Read the model definition and answer for the solid it produces. Units are mm, in the model's axes. A direction names the side the tool comes from. Coordinates: 2 decimals unless noted, no trailing zeros. Loops run counter-clockwise (first coordinate to the right, second up) from the corner with the lowest first, then second, coordinate; pieces in that order, holes last. Notation, with made-up numbers: (13, 56) - (32, 56) arc R21 cw to (32, 85) - close; hole circle Ø7 at (4, -30). An arc over 180 degrees is marked (long way). Use one line per item in the form item = value.
from build123d import *

# Parameters (mm, degrees)
SKETCH2_R           = 2.413
BOSS_EXTRUDE1_DEPTH = 57.15
CUT_EXTRUDE1_DEPTH  = 1.778
CHAMFER1_SIZE       = 0.428942381
FILLET1_R           = 0.381


with BuildPart() as part:
    # Sketch1 → Revolve1 (revolve)
    with BuildSketch(Plane.XZ):
        with BuildLine():
            Line((2.29235, 0), (0, 0))
            Line((0, 0), (0, -2.5654))
            Line((0, -2.5654), (4.5847, -2.5654))
            Line((4.5847, -2.5654), (4.5847, -2.0574))
            ThreePointArc((4.5847, -2.0574), (3.589105441, -0.860923645), (2.29235, 0))
        make_face()
    revolve(axis=Axis((0, 0, 0), (0, 0, -1)))

    # Sketch2 → Boss-Extrude1 (add)
    with BuildSketch(Plane(origin=(0, 0, -2.5654), x_dir=(-1, 0, 0), z_dir=(0, 0, -1))):
        Circle(SKETCH2_R)
    extrude(amount=BOSS_EXTRUDE1_DEPTH)

    # Sketch3 → Cut-Extrude1 (cut)
    with BuildSketch(Plane.XY):
        Polygon((1.5875, -0.916543552), (1.5875, 0.916543552), (0, 1.833087105), (-1.5875, 0.916543552), (-1.5875, -0.916543552), (0, -1.833087105), align=None)
    extrude(amount=-CUT_EXTRUDE1_DEPTH, mode=Mode.SUBTRACT)

    # Sketch4 → Cut-Revolve1 (revolve, cut)
    with BuildSketch(Plane.XZ):
        Polygon((1.5875, -1.778), (0, -1.778), (0, -2.694543552), align=None)
    revolve(axis=Axis((0, 0, -1.778), (0, 0, -1)), mode=Mode.SUBTRACT)

    # Chamfer1
    chamfer1_edges = [part.edges().sort_by_distance(p)[0] for p in [
        (2.413, 0, -59.7154),
    ]]
    chamfer(chamfer1_edges, length=CHAMFER1_SIZE)

    # Fillet1
    fillet1_edges = [part.edges().sort_by_distance(p)[0] for p in [
        (2.413, 0, -2.5654),
    ]]
    fillet(fillet1_edges, radius=FILLET1_R)


solid = part.part
Item 1: Find the intervals of material crossed by L1, parallel to Y at x = -0.75, z = -6; L2, parallel to Z at x = -3.5, y = -0.25, in increasing order.
Results below:
L1 = -2.29 to 2.29
L2 = -2.57 to -0.79
Item 2: For a pull along X with two mould halves and no side action, classify faces 4 (the flat face through (1.588, 0, -1)), 5 (the cylindrical face through (-3.64, 2.79, -2.31)), 6 (the flat face through (0, 3, -2.565)) as +X half, -X half, draft (parallel to the pull), parting line (faces both ways), or undercut.
Results below:
face_4 = undercut
face_5 = parting line
face_6 = draft
Item 3: The part is cut by section B-B on y = 3.5. Give the vertices of the cut face in (x, z).
Results below:
outline = (-2.96, -2.57) - (2.96, -2.57) - (2.96, -2.06) arc R4.08 ccw to (-2.96, -2.06) - close
Item 4: Each of these flat-tipped pins is pushed along its axis until it touches: P1, Ø4, axis at y = -2.5, z = -14.5, coming from the +X side; P2, Ø0.5, axis at y = 0, z = -1, coming from the +X side; P3, Ø2, axis at x = 2, z = -41.5, coming from the +Y side. Where does it stop, or does it pass through?
Results below:
P1 = 2.36
P2 = 3.98
P3 = 2.2
Item 5: The part is cut by section A-A on z = -22.5. Give the vertices of the cut face in (x, y), plus the area to 3 significant figures.
Results below:
outline = circle Ø4.83 at (0, 0)
area = 18.3 mm²
Item 6: The part is cut by section C-C on x = 4. Give the vertices of the cut face in (y, z).
Results below:
outline = (-2.24, -2.57) - (2.24, -2.57) - (2.24, -2.06) arc R3.59 ccw to (-2.24, -2.06) - close
Item 7: Which of the six approach directions +Z, -Z, +X, -X, +Y, -Y give full straight-line access (tool end or side, diameter ignored) to faces 1 (the flat face through (0.8, 1.37, -0.88)), 2 (the cylindrical face through (1.915, -1.468, -30.722)), 3 (the flat face through (0, -2, 0))?
Results below:
face_1 = +Z
face_2 = -Z
face_3 = +Z, +X, -X, +Y, -Y
